Solid Edge part; units mm, degrees
sketch "Sketch1" plane through (0, 0, 0) normal (0, 0, 1) x (1, 0, 0)
  circle A0 centre (0, 0) radius 2.725
extrude "Protrusion1" add sketch "Sketch1" against normal blind 3
sketch "Sketch2" plane through (0, 0, 0) normal (0, 0, 1) x (1, 0, 0)
  line L0 (-0.7, -1.2124) -> (-1.05, -0.6062)
  line L1 (-1.4, 0) -> (-1.05, -0.6062)
  line L2 (-1.4, 0) -> (-1.05, 0.6062)
  line L3 (-0.7, 1.2124) -> (-1.05, 0.6062)
  line L4 (-0.7, 1.2124) -> (0, 1.2124)
  line L5 (0.7, 1.2124) -> (0, 1.2124)
  line L6 (0.7, 1.2124) -> (1.05, 0.6062)
  line L7 (1.4, 0) -> (1.05, 0.6062)
  line L8 (1.4, 0) -> (1.05, -0.6062)
  line L9 (0.7, -1.2124) -> (1.05, -0.6062)
  line L10 (0.7, -1.2124) -> (0, -1.2124)
  line L11 (-0.7, -1.2124) -> (0, -1.2124)
extrude "ExtrudedCutout_1" cut sketch "Sketch2" against normal blind 1.45
sketch "Sketch3" plane through (0, 0, -3) normal (0, 0, -1) x (1, 0, 0)
  circle A0 centre (0, 0) radius 1.45
extrude "ExtrudedProtrusion_2" add sketch "Sketch3" along normal blind 30
properties material "Stainless steel"
For this review, take the finished solid that the model builds, in its own axes (mm). A direction names the side the tool comes from. Give positions to 0.01 mm unless a question says otherwise; leave off trailing zeros. Order: outer loops, then holes, each group sorted by start corner. A loop starts at its lowest first (then second) coordinate and runs counter-clockwise, first axis right, second up. Notation, with made-up numbers: (-12.75, -6.75) - (2.25, -6.75) arc R21 cw to (2.25, 14.25) - close; hole circle Ø10 at (4, 24). An arc over 180 degrees is marked (long way). Answer as a JSON object with one key per item and string values. Group by question number.
Item 1: Wall thickness on line 1 along Y through (x, z) = (-0.05, -13); line 2 along Z through (x, y) = (2.1, 1.6); line 3 along Z through (x, y) = (-0.4, -0.75): over which ranges is each line inside the solid? List them lowest first.
Item 2: Clearance check with a flat-ended pin moving along its axis: pin 1 Ø1 at (y, z) = (0, -28.5) entering from -X. State where the tip first meets the part, or that it passes through.
Item 3: Take a section at D-D on y = -1.8. Give the boundary of the cut face in (x, z).
Item 4: Draft analysis for pull direction Y (two halves, no side actions). For faces 1 (the flat face through (1.2, -1.2, -3)), 2 (the cylindrical face through (-1.45, 0.06, -17.79)), 3 (the flat face through (0, 0, -1.45)), 4 (the flat face through (1.055, 0.598, -0.715)), state which applies: pulls with the +Y half, pulls with the -Y half, needs draft (parallel to the pull), parting line crosses it, or undercut.
Item 5: Take a section at C-C on z = -29.5. Give the boundary of the cut face in (x, y), and give its area (3 significant figures).
Item 6: Take a section at A-A on x = 0. Give the boundary of the cut face in (y, z) (3 decimals), and give its area (3 significant figures).
Item 7: Machinability: for faces 5 (the flat face through (-1.055, -0.598, -0.715)), 6 (the cylindrical face through (2.6, 0.82, -1.48)), which of the approach directions +Z, -Z, +X, -X, +Y, -Y give a long, thin tool a straight path to every point of the face, cutting with its end or side? Answer none if there is none.
Item 8: Take a section at B-B on y = 0.4. Give the boundary of the cut face in (x, z), and give its area (3 significant figures).
Reported:
{
 "1": {"line 1": "-1.45 to 1.45", "line 2": "-3 to 0", "line 3": "-33 to -1.45"},
 "2": {"pin 1": "x = -1.45"},
 "3": {"outline": "(-2.05, -3) - (2.05, -3) - (2.05, 0) - (-2.05, 0) - close"},
 "4": {"face 1": "needs draft", "face 2": "parting line crosses it", "face 3": "undercut", "face 4": "undercut"},
 "5": {"outline": "circle Ø2.9 at (0, 0)", "area": "6.61 mm^2"},
 "6": {"outline": "(-2.725, -3) - (-1.45, -3) - (-1.45, -33) - (1.45, -33) - (1.45, -3) - (2.725, -3) - (2.725, 0) - (1.212, 0) - (1.212, -1.45) - (-1.212, -1.45) - (-1.212, 0) - (-2.725, 0) - close", "area": "99.8 mm^2"},
 "7": {"face 5": "+Z", "face 6": "+Z, -Z"},
 "8": {"outline": "(-2.7, -3) - (-1.39, -3) - (-1.39, -33) - (1.39, -33) - (1.39, -3) - (2.7, -3) - (2.7, 0) - (1.17, 0) - (1.17, -1.45) - (-1.17, -1.45) - (-1.17, 0) - (-2.7, 0) - close", "area": "96.4 mm^2"}
}
